Model file for the job. Use its own axes, mm. A direction names the side the tool comes from. Give positions to 0.01 mm unless a question says otherwise; leave off trailing zeros. Loops run counter-clockwise (first coordinate to the right, second up) from the corner with the lowest first, then second, coordinate; pieces in that order, holes last. Notation, with made-up numbers: M -2.75,-5 L 42.25,-5 A33 cw 42.25,32 Z; hole C 10.5,4 d4. An arc over 180 degrees is marked long. Answer in a Markdown table with one row per item.
```python
from build123d import *

# Parameters (mm, degrees)
F2_START      = -71.12
F2_DEPTH      = 88.9
F0_R          = 3.175
F0_R_2        = 1.9812
F0_R_3        = 4.7752
F3_DEPTH      = 25.4
F3_DEPTH_BACK = 25.4


with BuildPart() as f2:
    # F1 (on Front) → F2 (new body)
    with BuildSketch(Plane.XZ.offset(F2_START)):
        with BuildLine():
            Line((-8.6614, -53.2892), (-8.6614, -18.415))
            Line((-8.6614, -18.415), (-11.8364, -18.415))
            Line((-11.8364, -18.415), (-11.8364, -53.2892))
            ThreePointArc((-11.8364, -53.2892), (-10.3485024484, -56.8813024484), (-6.7564, -58.3692))
            Line((-6.7564, -58.3692), (0, -58.3692))
            Line((0, -58.3692), (6.7564, -58.3692))
            ThreePointArc((6.7564, -58.3692), (10.3485024484, -56.8813024484), (11.8364, -53.2892))
            Line((11.8364, -53.2892), (11.8364, -18.415))
            Line((11.8364, -18.415), (8.6614, -18.415))
            Line((8.6614, -18.415), (8.6614, -53.2892))
            ThreePointArc((8.6614, -53.2892), (8.1034384182, -54.6362384182), (6.7564, -55.1942))
            Line((6.7564, -55.1942), (0, -55.1942))
            Line((0, -55.1942), (-6.7564, -55.1942))
            ThreePointArc((-6.7564, -55.1942), (-8.1034384182, -54.6362384182), (-8.6614, -53.2892))
        make_face()
    extrude(amount=-F2_DEPTH)

    # F0 (on Right) → F3 (cut, two sides)
    with BuildSketch(Plane.YZ) as f3_sk:
        with Locations((77.47, -48.8442)):
            Circle(F0_R)
        with Locations((83.1596, -37.6936)):
            Circle(F0_R_2)
        with Locations((104.5718, -45.6692)):
            Circle(F0_R_2)
        with Locations((133.1468, -39.9542)):
            Circle(F0_R_3)
    extrude(amount=F3_DEPTH, mode=Mode.SUBTRACT)
    extrude(f3_sk.sketch, amount=-F3_DEPTH_BACK, mode=Mode.SUBTRACT)


solid = f2.part
```
Q1. Saw through at B-B (x = -9.75). Give the cut face in (y, z) (3 decimals).
Reported:
| item | result |
|---|---|
| outline | M 71.12,-57.393 L 160.02,-57.393 L 160.02,-18.415 L 71.12,-18.415 Z; hole C 77.47,-48.844 d6.35; hole C 83.16,-37.694 d3.962; hole C 104.572,-45.669 d3.962; hole C 133.147,-39.954 d9.55 |
Q2. Saw through at D-D (x = 3.75). Give the cut face in (y, z), and give its area (3 significant figures).
Reported:
| item | result |
|---|---|
| outline | M 71.12,-58.37 L 160.02,-58.37 L 160.02,-55.19 L 71.12,-55.19 Z |
| area | 282 mm² |
Q3. Drop flat-ended pins along their axis: pin 1 (5 mm diameter, centred on y = 77.47, z = -48.84, fed in from -X); pin 2 (4 mm diameter, centred on x = -2, y = 109, fed in from +Z); pin 3 (2 mm diameter, centred on x = -6.5, y = 98, fed in from +Z). Give the stop position or say it passes through.
Reported:
| item | result |
|---|---|
| pin 1 | through |
| pin 2 | z = -55.19 |
| pin 3 | z = -55.04 |
Q4. Probe probe 1 along X at (y, z) = (118, -50.5); probe 2 along Z at (x, y) = (-6.5, 102); probe 3 along Y at (x, z) = (-8.75, -43). List the from-to ranges inside material, lowest first.
Reported:
| item | result |
|---|---|
| probe 1 | -11.84 to -8.66, 8.66 to 11.84 |
| probe 2 | -58.37 to -55.19 |
| probe 3 | 71.12 to 129.47, 136.82 to 160.02 |
Q5. 3-axis set-ups, long thin cutter, end or side, ignore diameter. For faces 5 (the face through (-10, 115, -18.415)), 6 (the face through (8.12, 114.95, -54.62)): which of +Z, -Z, +X, -X, +Y, -Y reach the whole face in a straight line?
Reported:
| item | result |
|---|---|
| face 5 | +Z, +X, -X, +Y, -Y |
| face 6 | +Z, +Y, -Y |
Q6. Mould opens along X. For faces 1 (the face through (-10.39, 114.95, -56.84)), 2 (the face through (-10.23, 78.94, -51.66)), 3 (the face through (8.661, 115, -36)), 4 (the face through (11.836, 115, -36)) say: released by +X, released by -X, zero draft, split by the parting line, or undercut.
Reported:
| item | result |
|---|---|
| face 1 | released by -X |
| face 2 | zero draft |
| face 3 | undercut |
| face 4 | released by +X |
Q7. Saw through at A-A (y = 77.47). Give the cut face in (x, z) (3 decimals).
Reported:
| item | result |
|---|---|
| outline | M -11.836,-53.289 A5.08 ccw -6.756,-58.369 L 6.756,-58.369 A5.08 ccw 11.836,-53.289 L 11.836,-52.019 L 8.661,-52.019 L 8.661,-53.289 A1.905 cw 6.756,-55.194 L -6.756,-55.194 A1.905 cw -8.661,-53.289 L -8.661,-52.019 L -11.836,-52.019 Z; M -11.836,-45.669 L -8.661,-45.669 L -8.661,-18.415 L -11.836,-18.415 Z; M 8.661,-45.669 L 11.836,-45.669 L 11.836,-18.415 L 8.661,-18.415 Z |
Q8. Saw through at C-C (y = 152). Give the cut face in (x, z) (3 decimals).
Reported:
| item | result |
|---|---|
| outline | M -11.836,-53.289 A5.08 ccw -6.756,-58.369 L 6.756,-58.369 A5.08 ccw 11.836,-53.289 L 11.836,-18.415 L 8.661,-18.415 L 8.661,-53.289 A1.905 cw 6.756,-55.194 L -6.756,-55.194 A1.905 cw -8.661,-53.289 L -8.661,-18.415 L -11.836,-18.415 Z |
